Check sheet for the modelled part. Datum: model origin and axes. Units: mm. A direction names the side the tool comes from. Round coordinates to 2 decimals unless told otherwise and drop trailing zeros. Order: outer loops, then holes, each group sorted by start corner. A loop starts at its lowest first (then second) coordinate and runs counter-clockwise, first axis right, second up. Notation, with made-up numbers: (-11.75, 60.25) -> (4.25, 60.25) arc R24 ccw to (4.25, 85.25) -> close; hole circle Ø2 at (44.25, 9.5). An arc over 180 degrees is marked (long way). Answer in a Markdown table with one row per item. Add a question column.
1. Depth check by flat-ended pin: P1, Ø1, axis at y = -5, z = 2, coming from the +X side; P2, Ø2, axis at x = -1, y = -0.5, coming from the +Z side; P3, Ø1.5, axis at y = -2, z = -0.5, coming from the +X side; P4, Ø1.6, axis at x = -0.5, y = 2.5, coming from the -Z side. Enter the tip coordinate at first touch or a pass-through.
2. Material ranges on L1, parallel to Y at x = -2.5, z = 0.25; L2, parallel to Y at x = 0.75, z = 1; L3, parallel to X at y = 2.5, z = -0.5, recorded low to high. Write a range as from..to.
3. Sectioned sample at C-C, the plane z = -2.5. Record the boundary of the cut face in (x, y).
4. Sectioned sample at B-B, the plane y = -1.5. Record the boundary of the cut face in (x, z).
5. Sectioned sample at A-A, the plane x = 0. Record the boundary of the cut face in (y, z), then the cut area to 4 significant figures.
6. Access from +Z, -Z, +X, -X, +Y, -Y to the whole of each face (thin tool, end or side, straight path). Record for faces 1 (the cylindrical face through (0, -5, 2)), 2 (the flat face through (-2, 4, -1)), 3 (the flat face through (-1.724, 3.014, -1.014)).
7. Draft check along X on faces 4 (the flat face through (0, -10, 0)), 5 (the flat face through (1.74, 3.01, -0.99)), 6 (the flat face through (0, 3, 2)), 7 (the cylindrical face through (1.43, 1.97, -2.75)). Enter one of: +X half, -X half, draft (parallel to the pull), parting line (faces both ways), or undercut.
8. Sectioned sample at D-D, the plane y = 1.5. Record the boundary of the cut face in (x, z).
Solid Edge part; units mm, degrees
sketch "Sketch1" plane through (0, 0, 0) normal (0, -1, 0) x (1, 0, 0)
  circle A0 centre (0, 0) radius 3.1
extrude "Protrusion1" add sketch "Sketch1" against normal blind 4
sketch "Sketch2" plane through (0, 0, 0) normal (0, -1, 0) x (1, 0, 0)
  circle A0 centre (0, 0) radius 2
extrude "Protrusion2" add sketch "Sketch2" along normal blind 10
sketch "Sketch3" plane through (0, 4, 0) normal (0, 1, 0) x (-1, 0, 0)
  line L0 (1.1547, 2) -> (-1.1547, 2)
  line L1 (-1.1547, 2) -> (-2.3094, 0)
  line L2 (-2.3094, 0) -> (-1.1547, -2)
  line L3 (-1.1547, -2) -> (1.1547, -2)
  line L4 (1.1547, -2) -> (2.3094, 0)
  line L5 (2.3094, 0) -> (1.1547, 2)
extrude "Cutout1" cut sketch "Sketch3" against normal blind 2
chamfer "Chamfer1" distance 0.5 angle 45 1 edges at (-2, -10, 0)
properties part number "SOCKET2"
Answer key:
| question | item | result |
|---|---|---|
| 1 | P1 | stops at x = 1.32 |
| 1 | P2 | stops at z = 3.1 |
| 1 | P3 | stops at x = 2 |
| 1 | P4 | stops at z = -3.1 |
| 2 | L1 | y = 0..4 |
| 2 | L2 | y = -10..2 |
| 2 | L3 | x = -3.06..-2.02, 2.02..3.06 |
| 3 | outline | (-1.83, 0) -> (1.83, 0) -> (1.83, 4) -> (-1.83, 4) -> close |
| 4 | outline | circle Ø4 at (0, 0) |
| 5 | outline | (-10, -1.5) -> (-9.5, -2) -> (0, -2) -> (0, -3.1) -> (4, -3.1) -> (4, -2) -> (2, -2) -> (2, 2) -> (4, 2) -> (4, 3.1) -> (0, 3.1) -> (0, 2) -> (-9.5, 2) -> (-10, 1.5) -> close |
| 5 | area | 56.55 mm² |
| 6 | face 1 | -Y |
| 6 | face 2 | +Z, -Z, +X, -X, +Y |
| 6 | face 3 | +Y |
| 7 | face 4 | draft |
| 7 | face 5 | undercut |
| 7 | face 6 | undercut |
| 7 | face 7 | parting line |
| 8 | outline | circle Ø6.2 at (0, 0) |
